Autodesk Inventor part; units mm, degrees
ref_plane "YZ Plane" through (0, 0, 0) normal (1, 0, 0) x (0, 1, 0)
ref_plane "XZ Plane" through (0, 0, 0) normal (0, 1, 0) x (-1, 0, 0)
ref_plane "XY Plane" through (0, 0, 0) normal (0, 0, 1) x (1, 0, 0)
ref_plane "РабПлоскость1" through (0, 0, 0) normal (0, 0, 1) x (1, 0, 0)
sketch "Эскиз1" plane through (0, 0, 0) normal (0, 0, 1) x (1, 0, 0)
  line L0 (0, -90.9139) -> (0, -87.1819)
  line L1 (0, -75.9857) -> (0, -72.2537)
  line L2 (0, -72.2537) -> (3, -61.0575)
  line L3 (3, -61.0575) -> (0, -61.0575)
  line L4 (0, -61.0575) -> (0, -57.3255)
  line L5 (0, -57.3255) -> (3, -46.1293)
  line L6 (3, -46.1293) -> (0, -46.1293)
  line L7 (0, -46.1293) -> (0, -42.3973)
  line L8 (0, -42.3973) -> (3, -31.2011)
  line L9 (3, -31.2011) -> (0, -31.2011)
  line L10 (0, -31.2011) -> (0, -27.4691)
  line L11 (0, -27.4691) -> (3, -16.2729)
  line L12 (3, -16.2729) -> (0, -16.2729)
  line L13 (0, -16.2729) -> (0, -12.5409)
  line L14 (127.6, -12.5409) -> (0, -12.5409)
  line L15 (127.6, -57.3255) -> (124.6, -46.1293)
  line L16 (127.6, -61.0575) -> (127.6, -57.3255)
  line L17 (124.6, -61.0575) -> (127.6, -61.0575)
  line L18 (127.6, -72.2537) -> (124.6, -61.0575)
  line L19 (127.6, -75.9857) -> (127.6, -72.2537)
  line L20 (124.6, -75.9857) -> (127.6, -75.9857)
  line L21 (127.6, -87.1819) -> (124.6, -75.9857)
  line L22 (127.6, -90.9139) -> (127.6, -87.1819)
  line L23 (84.6, -94.6473) -> (84.6, -100.1704)
  line L24 (83.844, -94.6473) -> (84.6, -94.6473)
  line L25 (83.844, -94.6473) -> (84.844, -90.9152)
  line L26 (132.6, -90.9152) -> (84.844, -90.9152)
  line L27 (132.6, -90.9152) -> (134.6, -98.3793)
  line L28 (134.6, -98.3793) -> (134.6, 2.1319)
  line L29 (134.6, 2.1319) -> (-7, 2.1319)
  line L30 (-7, -98.3793) -> (-7, 2.1319)
  line L31 (-5, -90.9152) -> (-7, -98.3793)
  line L32 (127.6, -75.4591) -> (127.6, -90.9139)
  line L33 (0.2004, -110.9139) -> (127.4004, -110.9139)
  line L34 (127.4004, -110.9139) -> (127.4004, -70.9139)
  line L35 (127.4004, -70.9139) -> (0.2004, -70.9139)
  line L36 (0.2004, -70.9139) -> (0.2004, -110.9139)
  line L37 (0.2004, -110.9139) -> (127.4004, -70.9139) construction
  line L38 (127.4004, -110.9139) -> (0.2004, -70.9139) construction
  line L39 (51.0804, -92.9931) -> (38.3604, -115.0247)
  line L40 (38.3604, -115.0247) -> (12.9204, -115.0247)
  line L41 (12.9204, -115.0247) -> (0.2004, -92.9931)
  line L42 (0.2004, -70.9614) -> (63.8004, -70.9614)
  line L43 (38.3604, -70.9614) -> (51.0804, -92.9931)
  line L44 (-1, -89.7832) -> (-1, -91.3815)
  line L45 (0.2004, -92.9931) -> (5.8434, -102.7672)
  line L46 (63.8004, -70.9139) -> (63.8004, -110.9139)
  line L47 (51.0804, -92.9931) -> (63.8004, -92.9931)
  line L48 (0.2004, -92.9931) -> (-1, -90.9139)
  line L49 (5.9739, -102.9931) -> (45.3069, -102.9931)
  line L50 (-1, -90.9139) -> (0, -90.9139)
  line L51 (0, -90.9139) -> (0.2004, -90.9139)
  point P0 (0, 0)
  point P1 (63.8004, -90.9139)
  point P2 (25.6404, -92.9931)
  point P3 (5.9739, -102.9931)
  point P4 (0.3463, -70.9614)
  point P5 (0.2004, -71.5059)
  dimension "d0" = 127.6
  dimension "d1" = 127.2
  dimension "d2" = 40
  dimension "d3" = 50.88
  dimension "d4" = 0
  dimension "d5" = 1
  dimension "d6" = 25.44
  dimension "d7" = 10
extrude "Выдавливание1" add sketch "Эскиз1" along normal blind 1 contours L36 L42 L2 | L2 L42 L43 L39 L49 L41 L36 | L36 L48 L50 L51 | L42 L46 L47 L43
chamfer "Фаска1" distance 0.5 angle 45 4 edges at (0.2004, -70.9614, 0.5) (45.3069, -102.9931, 0.5) (5.9739, -102.9931, 0.5) (51.0804, -92.9931, 0.5)
sketch "Эскиз3" plane through (0.2004, -90.9139, 0) normal (-1, 0, 0) x (0, 0, 1)
  line L0 (-2.0003, -7.4654) -> (24.9316, 93.0458)
  line L1 (0, 19.4526) -> (1, 19.4526)
  line L2 (0, 19.4526) -> (0, 0)
  line L3 (0, 0) -> (1, 0)
  line L4 (1, 19.4526) -> (1, 0)
  line L5 (0, 0) -> (1, 0)
  point P0 (0, 90.9139)
  point P1 (1, 3.7321)
extrude "Выдавливание2" add sketch "Эскиз3" along normal blind 4 contours L0 L4 L3
sketch "Эскиз4" plane through (0, 0, 1) normal (0, 0, 1) x (1, 0, 0)
  line L0 (-1, -90.9139) -> (5.7239, -102.56)
  line L1 (0.2004, -90.9139) -> (-1, -90.9139)
  line L2 (-1, -90.9139) -> (-3.1547, -87.1819)
  line L3 (0.2004, -87.1819) -> (-3.7996, -87.1819)
  line L4 (-1, -90.9139) -> (-3.7996, -90.9139)
  line L5 (-3.7996, -90.9139) -> (-3.7996, -87.1819)
  point P0 (0, 0)
extrude "Выдавливание3" cut sketch "Эскиз4" against normal blind 4
sketch "Эскиз6" plane through (0, 0, 1) normal (0, 0, 1) x (1, 0, 0)
  line L0 (-3.1547, -87.1819) -> (5.7239, -102.56)
  line L1 (6.4739, -102.9931) -> (5.7239, -102.56)
  line L2 (6.4739, -102.9931) -> (44.8069, -102.9931)
  line L3 (45.5569, -102.56) -> (44.8069, -102.9931)
  line L4 (45.5569, -102.56) -> (50.8304, -93.4261)
  line L5 (51.5804, -92.9931) -> (50.8304, -93.4261)
  line L6 (51.5804, -92.9931) -> (63.8004, -92.9931)
  line L7 (63.8004, -92.9931) -> (63.8004, -70.9614)
  line L8 (63.8004, -70.9614) -> (0.7004, -70.9614)
  line L9 (0.2004, -71.4614) -> (0.7004, -70.9614)
  line L10 (0.2004, -71.4614) -> (0.2004, -87.1819)
  line L11 (0.2004, -87.1819) -> (-3.1547, -87.1819)
  line L12 (0.4004, -87.3819) -> (0.4004, -71.5442)
  line L13 (0.4004, -71.5442) -> (0.7832, -71.1614)
  line L14 (0.7832, -71.1614) -> (63.6004, -71.1614)
  line L15 (63.6004, -71.1614) -> (63.6004, -92.7931)
  line L16 (63.6004, -92.7931) -> (51.5268, -92.7931)
  line L17 (51.5268, -92.7931) -> (50.684, -93.2797)
  line L18 (50.684, -93.2797) -> (45.4105, -102.4136)
  line L19 (45.4105, -102.4136) -> (44.7533, -102.7931)
  line L20 (44.7533, -102.7931) -> (6.5275, -102.7931)
  line L21 (6.5275, -102.7931) -> (5.8703, -102.4136)
  line L22 (5.8703, -102.4136) -> (-2.8083, -87.3819)
  line L23 (-2.8083, -87.3819) -> (0.4004, -87.3819)
  line L24 (0.2004, -87.1819) -> (-3.1547, -87.1819)
  line L25 (0.2004, -87.1819) -> (0.4004, -87.1819)
  line L26 (0.7832, -71.1614) -> (0.9832, -70.9614)
  point P0 (0, 0)
  point P1 (0.8418, -70.9614)
  dimension "d20" = 0.2
extrude "Выдавливание5" cut sketch "Эскиз6" against normal blind 10 contours L10 L9 L8 L26 L13 L12 L25
sketch "Эскиз7" plane through (0, 0, 0) normal (0, 0, -1) x (-1, 0, 0)
  line L0 (-0.4004, -87.1819) -> (-0.4004, -71.5442)
  line L1 (-0.4004, -71.5442) -> (-0.9832, -70.9614)
  line L2 (-0.2004, -90.9139) -> (1, -90.9139)
  line L3 (-0.2004, -87.1819) -> (-0.2004, -90.9139)
  line L4 (-1.3004, -71.9614) -> (-1.3004, -88.1819)
  line L5 (-1.3004, -88.1819) -> (-1.2004, -88.1819)
  line L6 (-1.2004, -88.1819) -> (-1.2004, -91.9139)
  line L7 (-1.2004, -91.9139) -> (-0.7321, -91.9139)
  line L8 (-0.7321, -91.9139) -> (-6.4559, -101.828)
  line L9 (-6.4559, -101.828) -> (-6.7418, -101.9931)
  line L10 (-6.7418, -101.9931) -> (-44.5389, -101.9931)
  line L11 (-44.5389, -101.9931) -> (-44.8248, -101.828)
  line L12 (-44.8248, -101.828) -> (-50.0983, -92.694)
  line L13 (-50.0983, -92.694) -> (-51.3124, -91.9931)
  line L14 (-51.3124, -91.9931) -> (-62.8004, -91.9931)
  line L15 (-62.8004, -91.9931) -> (-62.8004, -71.9614)
  line L16 (-62.8004, -71.9614) -> (-1.3004, -71.9614)
  line L17 (-1.3004, -71.9614) -> (-62.8004, -81.9772) construction
  line L18 (-1.3807, -71.4679) -> (-62.8807, -81.4837)
  line L19 (-62.72, -82.4707) -> (-1.22, -72.4549)
  arc A0 (-1.22, -72.4549) -> (-1.3807, -71.4679) centre (-1.3004, -71.9614) ccw
  arc A1 (-62.8807, -81.4837) -> (-62.72, -82.4707) centre (-62.8004, -81.9772) ccw
  line L20 (-62.8004, -81.9772) -> (-1.2004, -91.9139) construction
  line L21 (-62.88, -82.4708) -> (-1.28, -92.4076)
  line L22 (-1.1207, -91.4203) -> (-62.7207, -81.4836)
  arc A2 (-62.7207, -81.4836) -> (-62.88, -82.4708) centre (-62.8004, -81.9772) ccw
  arc A3 (-1.28, -92.4076) -> (-1.1207, -91.4203) centre (-1.2004, -91.9139) ccw
  line L23 (-62.8004, -87.9931) -> (-1.2004, -87.9931) construction
  line L24 (-62.8004, -88.4931) -> (-1.2004, -88.4931)
  line L25 (-1.2004, -87.4931) -> (-62.8004, -87.4931)
  arc A4 (-62.8004, -87.4931) -> (-62.8004, -88.4931) centre (-62.8004, -87.9931) ccw
  arc A5 (-1.2004, -88.4931) -> (-1.2004, -87.4931) centre (-1.2004, -87.9931) ccw
  line L26 (-62.8004, -75.9614) -> (-1.3004, -75.9614) construction
  line L27 (-62.8004, -76.4614) -> (-1.3004, -76.4614)
  line L28 (-1.3004, -75.4614) -> (-62.8004, -75.4614)
  arc A6 (-62.8004, -75.4614) -> (-62.8004, -76.4614) centre (-62.8004, -75.9614) ccw
  arc A7 (-1.3004, -76.4614) -> (-1.3004, -75.4614) centre (-1.3004, -75.9614) ccw
  line L29 (-62.8004, -81.9772) -> (-1.3004, -81.9772) construction
  line L30 (-62.8004, -82.4772) -> (-1.3004, -82.4772)
  line L31 (-1.3004, -81.4772) -> (-62.8004, -81.4772)
  arc A8 (-62.8004, -81.4772) -> (-62.8004, -82.4772) centre (-62.8004, -81.9772) ccw
  arc A9 (-1.3004, -82.4772) -> (-1.3004, -81.4772) centre (-1.3004, -81.9772) ccw
  line L32 (-0.2004, -87.1819) -> (-0.4004, -87.1819)
  line L33 (-63.8004, -70.9614) -> (-0.9832, -70.9614)
  line L34 (-63.8004, -92.9931) -> (-63.8004, -70.9614)
  line L35 (-51.5804, -92.9931) -> (-63.8004, -92.9931)
  line L36 (-50.8304, -93.4261) -> (-51.5804, -92.9931)
  line L37 (-45.5569, -102.56) -> (-50.8304, -93.4261)
  line L38 (-44.8069, -102.9931) -> (-45.5569, -102.56)
  line L39 (-6.4739, -102.9931) -> (-44.8069, -102.9931)
  line L40 (-5.7239, -102.56) -> (-6.4739, -102.9931)
  line L41 (1, -90.9139) -> (-5.7239, -102.56)
  point P0 (0, 0)
  point P1 (-32.0504, -76.9693)
  point P2 (-32.0004, -86.9456)
  point P3 (-62.8004, -81.4706)
  point P4 (-4.411, -71.9614)
  point P5 (-0.9953, -92.37)
  point P6 (-62.8004, -82.4837)
  point P7 (-1.3004, -72.468)
  point P8 (-59.6753, -81.9749)
  point P9 (-1.2004, -91.4075)
  point P10 (-32.0004, -87.9931)
  point P11 (-32.0504, -75.9614)
  point P12 (-32.0504, -81.9772)
  point P13 (-25.9019, -75.4614)
  point P14 (-19.6807, -75.4614)
  point P15 (-1.2004, -88.4931)
  point P16 (-19.2676, -88.4931)
  point P17 (-32.0422, -76.4614)
  point P18 (-56.6197, -81.4772)
  point P19 (-1.3004, -76.4614)
  point P20 (-25.821, -76.4614)
  point P21 (-1.3004, -82.4772)
  point P22 (-56.5611, -82.4772)
  point P23 (-25.4668, -87.4931)
  point P24 (-1.3004, -87.4931)
  point P25 (-31.7461, -87.4931)
  point P26 (-25.5469, -88.4931)
  dimension "d24" = 1
  dimension "d25" = 1
  dimension "d28" = 1
  dimension "d30" = 1
  dimension "d32" = 1
extrude "Выдавливание6" [suppressed]
mirror "Зеркальное отражение2" about plane through (63.8004, -92.9931, 0) normal (1, 0, 0)
properties part number "Пластина"
Read the model definition and answer for the solid it produces. Units are mm, in the model's axes. A direction names the side the tool comes from. Give positions to 0.01 mm unless a question says otherwise; leave off trailing zeros. Write each loop counter-clockwise with the first axis right and the second up, starting at its lowest first coordinate (ties: lowest second). Pieces come first, ordered by that corner, then holes. Notation, with made-up numbers: (-38.5, 47.5) -> (9.5, 47.5) arc R26 ccw to (9.5, 74.5) -> close; hole circle Ø8 at (-26.5, 55). An arc over 180 degrees is marked (long way). Answer as a JSON object with one key per item and string values. Group by question number.
1) Find section A-A (z = 0.3). Write down the section's boundary in (x, y), and give its area (3 significant figures).
2) Find section B-B (y = -77). Write down the section's boundary in (x, z), and give its area (3 significant figures).
3) The mould has two halves that part along X. Classify faces 1 (the flat face through (63, -87, 0)), 2 (the flat face through (79.444, -98.057, 0.493)): +X half, -X half, draft (parallel to the pull), parting line (faces both ways), or undercut.
4) Find section C-C (x = 62.5). Write down the section's boundary in (y, z).
5) A tool of negligible diameter and unlimited length cuts with its end or side. For faces 3 (the flat face through (-1.081, -88.659, 0.604)), 4 (the flat face through (48.23, -97.93, 0.49)), 5 (the flat face through (128.682, -88.607, 0.618)), from which of +Z, -Z, +X, -X, +Y, -Y can it reach the whole face along a straight path? Write none if from no direction.
6) Each of these flat-tipped pins is pushed along its axis until it touches: P1, Ø0.5, axis at x = 69, z = 0.5, coming from the -Y side; P2, Ø0.5, axis at y = -89, z = 0.5, coming from the +X side. Where does it stop, or does it pass through?
7) Consider L1, parallel to Y at x = 58, z = 0.7; L2, parallel to X at y = -96, z = 0.5; L3, parallel to X at y = -81, z = 0.25. Determine where each line is inside the solid, lowest interval first. Write a range as from..to.
Values follow:
{
 "1": {"outline": "(-1.65, -89.79) -> (-1, -90.91) -> (0.2, -92.99) -> (5.72, -102.56) -> (6.47, -102.99) -> (44.81, -102.99) -> (45.56, -102.56) -> (50.83, -93.43) -> (51.58, -92.99) -> (76.02, -92.99) -> (76.77, -93.43) -> (82.04, -102.56) -> (82.79, -102.99) -> (121.13, -102.99) -> (121.88, -102.56) -> (127.4, -92.99) -> (128.6, -90.91) -> (129.25, -89.79) -> (127.4, -89.79) -> (127.4, -87.18) -> (127.2, -87.18) -> (127.2, -71.54) -> (126.62, -70.96) -> (0.98, -70.96) -> (0.4, -71.54) -> (0.4, -87.18) -> (0.2, -87.18) -> (0.2, -89.79) -> close", "area": "3,700 mm2"},
 "2": {"outline": "(0.4, 0) -> (127.2, 0) -> (127.2, 1) -> (0.4, 1) -> close", "area": "127 mm2"},
 "3": {"face 1": "draft", "face 2": "undercut"},
 "4": {"outline": "(-92.99, 0) -> (-70.96, 0) -> (-70.96, 1) -> (-92.99, 1) -> close"},
 "5": {"face 3": "-Z, -X, +Y", "face 4": "+Z, -Z, -Y", "face 5": "-Z, +X, +Y"},
 "6": {"P1": "stops at y = -92.99", "P2": "stops at x = 129.84"},
 "7": {"L1": "y = -92.99..-70.96", "L2": "x = 1.94..49.34, 78.26..125.66", "L3": "x = 0.4..127.2"}
}
